Could you check a few things on this model? Use its own coordinates, in mm. Give positions to 0.01 mm unless a question says otherwise; leave off trailing zeros. Write each loop counter-clockwise with the first axis right and the second up, starting at its lowest first coordinate (ties: lowest second). Pieces come first, ordered by that corner, then holes. Notation, with made-up numbers: M 74.25,48 L 99.25,48 A28 cw 99.25,83 Z; hole C 9.25,-24 d9. An arc over 180 degrees is marked long. Answer as CSV lines item,"result". Start each with the question number.
Autodesk Inventor part; units mm, degrees
ref_plane "YZ Plane" through (0, 0, 0) normal (1, 0, 0) x (0, 1, 0)
ref_plane "XZ Plane" through (0, 0, 0) normal (0, 1, 0) x (-1, 0, 0)
ref_plane "XY Plane" through (0, 0, 0) normal (0, 0, 1) x (1, 0, 0)
sketch "Sketch1" plane through (0, 0, 0) normal (0, 0, 1) x (1, 0, 0)
  circle A0 centre (0, 0) radius 16.25
  circle A1 centre (0, 0) radius 13.5 construction
  circle A2 centre (0, 0) radius 11 construction
  line L0 (0, 13.5) -> (0, 0) construction
  line L1 (0, 0) -> (9.5263, 5.5) construction
  dimension "d2" = 22
  dimension "d0" = 32.5
  dimension "d1" = 27
  dimension "d3" = 60
extrude "Extrusion1" add sketch "Sketch1" along normal blind 5
hole "Hole1" at (0, 13.5, 0) at (9.5263, 5.5, 0) direction (0, 0, 1) diameter 3.242 depth 5
pattern_circular "Circular Pattern1" count 3 over 360 about axis through (0, 0, 0) along (0, 0, 1) of "Hole1"
chamfer "Chamfer1" distance 0.2 angle 45 2 edges at (-16.25, 0, 5) (-16.25, 0, 0)
equation "\"d2\" = holesid"
equation "\"holesid\" = 22"
properties part number "flange-adapter" material "Stainless Steel"
1. Please list where these lines run through material, in increasing order: line 1 (X direction, y = -6.75, z = 2.55); line 2 (Y direction, x = 0, z = 2.05); line 3 (X direction, y = 5.5, z = 1.3).
2. Imagine slicing it at C-C, the plane y = 5.5. State how many separate pieces and enclosed holes the cut face has, plus the area to 3 significant figures.
3. Will these pins go through, and if not, where does the flat tip stop? P1, Ø5, axis at x = 0, y = -11, coming from the -Z side; P2, Ø2.5, axis at x = -9.53, y = 5.5, coming from the -Z side; P3, Ø2, axis at x = -2.5, z = 3, coming from the +Y side.
4. Imagine slicing it at A-A, the plane x = 0. Please give me the cut outline in (y, z).
5. Imagine slicing it at B-B, the plane z = 2.2. Please give me the cut outline in (x, y).
6. Thinking about a two-plate mould opening in Y: for faces 1 (the flat face through (0, 0, 5)), 2 (the cylindrical face through (7.92, 5.29, 2.54)), 3 (the cylindrical face through (15.5, -4.88, 2.47)), which applies, pulls with the +Y half, pulls with the -Y half, needs draft (parallel to the pull), parting line crosses it, or undercut?
Solutions:
1,line 1,"-14.78 to -13.31, -10.07 to 10.07, 13.31 to 14.78"
1,line 2,"-16.25 to -12.62, -9.38 to 11.88, 15.12 to 16.25"
1,line 3,"-15.29 to -11.15, -7.91 to 7.91, 11.15 to 15.29"
2,separate pieces,"3"
2,enclosed holes,"0"
2,area,"120 mm²"
3,P1,"z = 0"
3,P2,"through"
3,P3,"y = 16.18"
4,outline,"M -16.25,0.2 L -16.05,0 L -12.62,0 L -12.62,5 L -16.05,5 L -16.25,4.8 Z; M -9.38,0 L 11.88,0 L 11.88,5 L -9.38,5 Z; M 15.12,0 L 16.05,0 L 16.25,0.2 L 16.25,4.8 L 16.05,5 L 15.12,5 Z"
5,outline,"C 0,0 d32.5; hole C -11.69,-6.75 d3.24; hole C -9.53,5.5 d3.24; hole C 0,-11 d3.24; hole C 0,13.5 d3.24; hole C 9.53,5.5 d3.24; hole C 11.69,-6.75 d3.24"
6,face 1,"needs draft"
6,face 2,"undercut"
6,face 3,"parting line crosses it"
